Source: CAD feature listing. Evaluate the final solid. Frame: model axes, mm. A direction names the side the tool comes from. Coordinates: 2 decimals unless noted, no trailing zeros. Write each loop counter-clockwise with the first axis right and the second up, starting at its lowest first coordinate (ties: lowest second). Pieces come first, ordered by that corner, then holes. Notation, with made-up numbers: (9, 15.25) -> (21, 15.25) arc R18 cw to (21, 39.25) -> close; hole circle Ø3 at (36.5, 42.25). An arc over 180 degrees is marked (long way). One line per item, written item: value. Start each with the question number.
1. Access query for faces 4 (the flat face through (1, 45, 136.959)), 5 (the flat face through (0.8, 22.5, 141.4)), 6 (the cylindrical face through (3.99, 24.26, 141.38)), 7 (the flat face through (2, 67.561, 141)), 8 (the flat face through (2, 45, 147.259)). Directions: +Z, -Z, +X, -X, +Y, -Y. A direction counts if a zero-diameter tool reaches every point of the face in a straight line with its end or side. Return the directions, or none.
2. First-contact query: P1, Ø1.6, axis at x = 2, z = 141.5, coming from the +Y side; P2, Ø0.6, axis at x = 4, y = 40, coming from the +Z side; P3, Ø4, axis at y = 32, z = 144.5, coming from the +X side; P4, Ø1, axis at x = 2, y = 62.5, coming from the +Z side. Flat tips, straight axial feed; report the tip coordinate or a pass-through.
3. Section query B-B, the plane y = 54.5. State how many separate pieces and enclosed holes the cut face has, and give its area (3 significant figures).
4. Line query: line 1 (Y direction, x = 2.2, z = 140.25); line 2 (Z direction, x = 3.1, y = 40.5); line 3 (X direction, y = 49, z = 135). Output: solid intervals per line, ascending.
5. Mould query, pull axis Y, two halves, no side actions, for faces 1 (the flat face through (3, 43, 135)), 2 (the flat face through (0.78, 67.315, 141.442)), 3 (the flat face through (4, 45, 137.477)). Classes: released by +Y, released by -Y, zero draft, split by the parting line, or undercut.
6. Section query A-A, the plane x = 2. Output: boundary loops of the cut face in (y, z), and give its area (3 significant figures).
from build123d import *

# Parameters (mm, degrees)
SKETCH_1_W          = 11.8
SKETCH_1_H          = 45.3
SKETCH_1_W_2        = 8.8
SKETCH_1_H_2        = 42.3
EXTRUDE_1_DEPTH     = 3
EXTRUDE_2_DEPTH     = 2
EXTRUDE_2_TAPER     = 30
CUT_EXTRUDE_1_REACH = 4
CHAMFER_1_SIZE      = 0.5
CHAMFER_1_SIZE2     = 1.538841769


with BuildPart() as part:
    # 草图1 → 凸台-拉伸1 (new body)
    with BuildSketch(Plane(origin=(0, 0, 0), x_dir=(0, 0, -1), z_dir=(1, 0, 0))):
        with Locations((-141.359181517, 44.911156128)):
            Rectangle(SKETCH_1_W, SKETCH_1_H)
        with Locations((-141.359181517, 44.911156128)):
            Rectangle(SKETCH_1_W_2, SKETCH_1_H_2, mode=Mode.SUBTRACT)
    extrude(amount=EXTRUDE_1_DEPTH)

    # 草图2 → 凸台-拉伸2 (add)
    with BuildSketch(Plane(origin=(3, 0, 0), x_dir=(0, 0, -1), z_dir=(1, 0, 0))):
        with BuildLine():
            Line((-146.259181517, 20.261156128), (-136.459181517, 20.261156128))
            ThreePointArc((-136.459181517, 20.261156128), (-134.337861173, 21.139835784), (-133.459181517, 23.261156128))
            Line((-133.459181517, 23.261156128), (-133.459181517, 66.561156128))
            ThreePointArc((-133.459181517, 66.561156128), (-134.337861173, 68.682476471), (-136.459181517, 69.561156128))
            Line((-136.459181517, 69.561156128), (-146.259181517, 69.561156128))
            ThreePointArc((-146.259181517, 69.561156128), (-148.38050186, 68.682476471), (-149.259181517, 66.561156128))
            Line((-149.259181517, 66.561156128), (-149.259181517, 23.261156128))
            ThreePointArc((-149.259181517, 23.261156128), (-148.38050186, 21.139835784), (-146.259181517, 20.261156128))
        make_face()
    extrude(amount=EXTRUDE_2_DEPTH, taper=EXTRUDE_2_TAPER)

    # 草图3 → 切除-拉伸1 (cut, up to next)
    with BuildSketch(Plane.ZY.offset(-3), mode=Mode.PRIVATE) as cut_extrude_1_sk1:
        with BuildLine():
            Line((145.241468338, 64.561156128), (145.241468338, 25.261156128))
            ThreePointArc((145.241468338, 25.261156128), (144.241468338, 24.261156128), (143.241468338, 25.261156128))
            Line((143.241468338, 25.261156128), (143.241468338, 64.561156128))
            ThreePointArc((143.241468338, 64.561156128), (144.241468338, 65.561156128), (145.241468338, 64.561156128))
        make_face()
    cut_extrude_1_tool1 = extrude(cut_extrude_1_sk1.sketch, amount=-CUT_EXTRUDE_1_REACH, mode=Mode.PRIVATE) & part.part
    add(cut_extrude_1_tool1.solids().sort_by_distance((3, 44.911156, 144.241468))[0], mode=Mode.SUBTRACT)
    # 草图3 → 切除-拉伸1 (cut, up to next)
    with BuildSketch(Plane.ZY.offset(-3), mode=Mode.PRIVATE) as cut_extrude_1_sk2:
        with BuildLine():
            Line((142.359181517, 64.561156128), (142.359181517, 25.261156128))
            ThreePointArc((142.359181517, 25.261156128), (141.359181517, 24.261156128), (140.359181517, 25.261156128))
            Line((140.359181517, 25.261156128), (140.359181517, 64.561156128))
            ThreePointArc((140.359181517, 64.561156128), (141.359181517, 65.561156128), (142.359181517, 64.561156128))
        make_face()
    cut_extrude_1_tool2 = extrude(cut_extrude_1_sk2.sketch, amount=-CUT_EXTRUDE_1_REACH, mode=Mode.PRIVATE) & part.part
    add(cut_extrude_1_tool2.solids().sort_by_distance((3, 44.911156, 141.359182))[0], mode=Mode.SUBTRACT)
    # 草图3 → 切除-拉伸1 (cut, up to next)
    with BuildSketch(Plane.ZY.offset(-3), mode=Mode.PRIVATE) as cut_extrude_1_sk3:
        with BuildLine():
            Line((139.476894696, 64.561156128), (139.476894696, 25.261156128))
            ThreePointArc((139.476894696, 25.261156128), (138.476894696, 24.261156128), (137.476894696, 25.261156128))
            Line((137.476894696, 25.261156128), (137.476894696, 64.561156128))
            ThreePointArc((137.476894696, 64.561156128), (138.476894696, 65.561156128), (139.476894696, 64.561156128))
        make_face()
    cut_extrude_1_tool3 = extrude(cut_extrude_1_sk3.sketch, amount=-CUT_EXTRUDE_1_REACH, mode=Mode.PRIVATE) & part.part
    add(cut_extrude_1_tool3.solids().sort_by_distance((3, 44.911156, 138.476895))[0], mode=Mode.SUBTRACT)

    # 倒角1
    chamfer_1_edges = [part.edges().sort_by_distance(p)[0] for p in [
        (0, 67.561156128, 141.359181517),
        (0, 44.911156128, 135.459181517),
        (0, 22.261156128, 141.359181517),
        (0, 44.911156128, 147.259181517),
    ]]
    chamfer_1_side = [part.faces().sort_by_distance(p)[0] for p in [
        (0, 67.093039689, 141.359181517),
    ]]
    chamfer(chamfer_1_edges, length=CHAMFER_1_SIZE, length2=CHAMFER_1_SIZE2, reference=chamfer_1_side[0])


solid = part.part
Computed values:
1. face 4: -X
1. face 5: +Z, -Z, -X, -Y
1. face 6: +X, -X
1. face 7: +Z, -Z, -X, +Y
1. face 8: +Z, -X, +Y, -Y
2. P1: stops at y = 67.56
2. P2: stops at z = 148.86
2. P3: stops at x = 5
2. P4: stops at z = 147.26
3. separate pieces: 4
3. enclosed holes: 0
3. area: 25.5 mm²
4. line 1: y = 22.26 to 23.76, 66.06 to 67.56
4. line 2: z = 133.52 to 137.48, 139.48 to 140.36, 142.36 to 143.24, 145.24 to 149.2
4. line 3: x = 3 to 5
5. face 1: zero draft
5. face 2: released by +Y
5. face 3: undercut
6. outline: (22.26, 135.46) -> (67.56, 135.46) -> (67.56, 147.26) -> (22.26, 147.26) -> close; hole (23.76, 136.96) -> (66.06, 136.96) -> (66.06, 145.76) -> (23.76, 145.76) -> close
6. area: 162 mm²
